Geometry check sheet. Reference: the model listing, model coordinates, mm. Face numbers are marked on the shaded views. A direction names the side the tool comes from. Round coordinates to 2 decimals unless told otherwise and drop trailing zeros. Order: outer loops, then holes, each group sorted by start corner. A loop starts at its lowest first (then second) coordinate and runs counter-clockwise, first axis right, second up.
(1) Cross-section at D-D on x = 24.5. Enter the section's corners in (y, z), and give its area (3 significant figures).
(2) Set-up check for the marked faces 1, 2, 3 and 4: record each of +Z, -Z, +X, -X, +Y, -Y from which the full face is reachable in a straight line by a thin tool's end or side.
(3) Gauge pin test, flat ends, axial feed: P1, Ø6.5, axis at x = 8, z = -18, coming from the -Y side; P2, Ø10.5, axis at y = 21.5, z = -8, coming from the -X side; P3, Ø8, axis at x = 6.5, z = -5.5, coming from the +Y side; P4, Ø10.5, axis at x = 45.5, y = 13, coming from the +Z side. Record the tip position at first contact, or that the pin passes through.
(4) Cross-section at C-C on z = -3. Enter the section's corners in (x, y).
(5) Cross-section at B-B on x = 52. Enter the section's corners in (y, z), and give its area (3 significant figures).
(6) Thickness scan on L1, parallel to X at y = -3, z = -3; L2, parallel to Z at x = 42, y = 18; L3, parallel to X at y = 52, z = -7.5. Record the ranges inside material, lowest first.
(7) Draft check along Z on the marked faces 5, 6, 7 and 8. Enter one of: pulls with the +Z half, pulls with the -Z half, needs draft (parallel to the pull), parting line crosses it, or undercut.
(8) Cross-section at A-A on y = 8. Enter the section's corners in (x, z), and give its area (3 significant figures).
Autodesk Inventor part; units mm, degrees
ref_plane "YZ Plane" through (0, 0, 0) normal (1, 0, 0) x (0, 1, 0)
ref_plane "XZ Plane" through (0, 0, 0) normal (0, 1, 0) x (-1, 0, 0)
ref_plane "XY Plane" through (0, 0, 0) normal (0, 0, 1) x (1, 0, 0)
sketch "Skizze4" plane through (0, 0, 0) normal (0, 0, 1) x (1, 0, 0)
  line L0 (0, 0) -> (0, 2)
  line L1 (0, 2) -> (22, 2)
  line L2 (22, 2) -> (22, -6)
  line L3 (22, -6) -> (37, -6)
  line L4 (37, -6) -> (37, 74)
  line L5 (37, 74) -> (62, 74)
  line L6 (62, 74) -> (62, -8)
  line L7 (62, 74) -> (144, 74) construction
  line L8 (62, -8) -> (21, -8)
  line L9 (21, -8) -> (21, 0)
  line L10 (21, 0) -> (0, 0)
  dimension "d2" = 2
  dimension "d3" = 22
  dimension "d4" = 8
  dimension "d5" = 15
  dimension "d6" = 80
  dimension "d7" = 25
  dimension "d8" = 82
  dimension "d9" = 90
  dimension "d10" = 41
extrude "Extrusion3" add sketch "Skizze4" against normal blind 25
sketch "Skizze7" plane through (37, 74, 0) normal (0, 1, 0) x (1, 0, 0)
  line L0 (2, 2) -> (23, 2)
  line L1 (23, 2) -> (23, 23)
  line L2 (23, 23) -> (2, 23)
  line L3 (2, 23) -> (2, 2)
  point P0 (-37, 0)
  dimension "d19" = 21
  dimension "d20" = 21
extrude "Extrusion4" cut sketch "Skizze7" against normal blind 100
properties part number "flexibler_standfuß_v0.2"
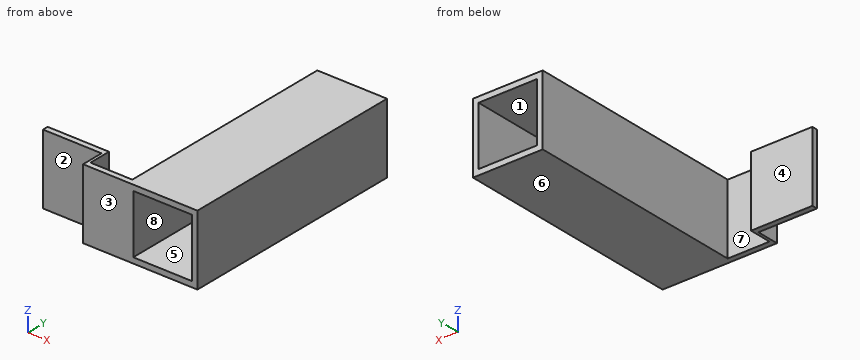
Found:
1. outline: (-8, -25) - (-6, -25) - (-6, 0) - (-8, 0) - close
1. area: 50.0 mm2
2. face 1: +Y, -Y
2. face 2: +Z, -Z, -X, -Y
2. face 3: +Z, -Z, +X, -X, -Y
2. face 4: +Z, -Z, -X, +Y
3. P1: stops at y = 0
3. P2: stops at x = 37
3. P3: stops at y = 2
3. P4: stops at z = 0
4. outline: (0, 0) - (21, 0) - (21, -8) - (39, -8) - (39, 74) - (37, 74) - (37, -6) - (22, -6) - (22, 2) - (0, 2) - close; (60, -8) - (62, -8) - (62, 74) - (60, 74) - close
5. outline: (-8, -25) - (74, -25) - (74, -23) - (-8, -23) - close; (-8, -2) - (74, -2) - (74, 0) - (-8, 0) - close
5. area: 328 mm2
6. L1: x = 21 to 22, 37 to 39, 60 to 62
6. L2: z = -25 to -23, -2 to 0
6. L3: x = 37 to 39, 60 to 62
7. face 5: undercut
7. face 6: pulls with the -Z half
7. face 7: needs draft
7. face 8: undercut
8. outline: (37, -25) - (62, -25) - (62, 0) - (37, 0) - close; hole (39, -23) - (60, -23) - (60, -2) - (39, -2) - close
8. area: 184 mm2
